Can you work these out from the model? Positions are in its coordinate system, mm. Round coordinates to 2 decimals unless told otherwise and drop trailing zeros. Write each loop counter-clockwise with the first axis right and the second up, starting at its lowest first coordinate (ties: lowest second). Pieces come first, ordered by that corner, then holes. Notation, with made-up numbers: (69.25, 15.5) -> (105.25, 15.5) arc R30 ccw to (105.25, 39.5) -> close; hole circle Ø1 at (73, 65). An arc over 180 degrees is marked (long way). Write item = value, one per line. Start each with the question number.
1) Imagine slicing it at C-C, the plane x = -71. Please give me the cut outline in (y, z), then the cut area to 3 significant figures.
2) Imagine slicing it at A-A, the plane y = 1. State how many separate pieces and enclosed holes the cut face has, then the cut area to 3 significant figures.
3) Imagine slicing it at B-B, the plane x = 10. Please give me the cut outline in (y, z).
4) If I drill on line 1 (Z direction, x = 80, y = 0.4); line 2 (X direction, y = 0.2, z = 38.5), over which ranges is the centre line in solid material (lowest first)?
5) I'm going to push flat-ended pins straight in: pin 1 (8 mm diameter, centred on x = -59, z = -58.5, fed in from -Y); pin 2 (0.6 mm diameter, centred on y = 1, z = 94, fed in from -X); pin 3 (1 mm diameter, centred on x = 0, y = 1, fed in from +Z); pin 4 (3 mm diameter, centred on x = 38.5, z = -38.5, fed in from +Y). Where does each tip first touch, or does it pass through?
from build123d import *

# Parameters (mm, degrees)
BOSS_EXTRUDE1_DEPTH     = 2
CUT_EXTRUDE1_DEPTH      = 139.261075506
CUT_EXTRUDE1_DEPTH_BACK = 139.261075506
SKETCH2_R               = 1
CHAMFER1_SIZE           = 1.5


with BuildPart() as part:
    # Sketch1 → Boss-Extrude1 (new body)
    with BuildSketch(Plane(origin=(0, 0, 0), x_dir=(1, 0, 0), z_dir=(0, 1, 0))):
        Polygon((5.75, -96.75), (61.746519787, -96.75), (61.746519787, -89.753578842), (73.246519787, -89.753578842), (73.246519787, -96.75), (96.75, -96.75), (96.75, -92.65), (91.75, -92.65), (91.75, -82.15), (96.75, -82.15), (96.75, 96.75), (23.65, 96.75), (23.65, 88.15), (-23.65, 88.15), (-23.65, 96.75), (-96.75, 96.75), (-96.75, -85.05), (-98.75, -85.05), (-98.75, -89.75), (-96.75, -89.75), (-96.75, -96.75), (-73.246519787, -96.75), (-73.246519787, -89.753578842), (-61.746519787, -89.753578842), (-61.746519787, -96.75), (-5.75, -96.75), (-5.75, -89.753578842), (5.75, -89.753578842), align=None)
    extrude(amount=BOSS_EXTRUDE1_DEPTH)

    # Sketch2 → Cut-Extrude1 (cut, two sides: drawn at the far end of the back side and taken through both)
    with BuildSketch(Plane.XZ.offset(-CUT_EXTRUDE1_DEPTH_BACK)):
        with Locations(Location((80, 80, 0), (0, 0, 270))):
            Circle(SKETCH2_R)
        with Locations(Location((-80, 80, 0), (0, 0, 270))):
            Circle(SKETCH2_R)
        with Locations(Location((-38.5, 38.5, 0), (0, 0, 270))):
            Circle(SKETCH2_R)
        with Locations(Location((38.5, 38.5, 0), (0, 0, 270))):
            Circle(SKETCH2_R)
        with Locations(Location((80, -80, 0), (0, 0, 270))):
            Circle(SKETCH2_R)
        with Locations(Location((-80, -80, 0), (0, 0, 270))):
            Circle(SKETCH2_R)
        with Locations(Location((38.5, -38.5, 0), (0, 0, 270))):
            Circle(SKETCH2_R)
        with Locations(Location((-38.5, -38.5, 0), (0, 0, 270))):
            Circle(SKETCH2_R)
    extrude(amount=CUT_EXTRUDE1_DEPTH + CUT_EXTRUDE1_DEPTH_BACK, mode=Mode.SUBTRACT)

    # Chamfer1
    chamfer1_edges = [part.edges().sort_by_distance(p)[0] for p in [
        (-80, 2, 81),
        (-38.5, 2, 39.5),
        (38.5, 2, 39.5),
        (80, 2, -79),
        (-38.5, 2, -37.5),
        (38.5, 2, -37.5),
        (-80, 2, -79),
        (80, 2, 81),
    ]]
    chamfer(chamfer1_edges, length=CHAMFER1_SIZE)


solid = part.part
Reported:
q1.outline = (0, -96.75) -> (2, -96.75) -> (2, 89.75) -> (0, 89.75) -> close
q1.area = 373 mm²
q2.separate_pieces = 1
q2.enclosed_holes = 8
q2.area = 36,700 mm²
q3.outline = (0, -88.15) -> (2, -88.15) -> (2, 96.75) -> (0, 96.75) -> close
q4.line_1 = -96.75 to -81, -79 to 79, 81 to 96.75
q4.line_2 = -96.75 to -39.5, -37.5 to 37.5, 39.5 to 96.75
q5.pin_1 = 0
q5.pin_2 = -96.75
q5.pin_3 = 89.75
q5.pin_4 = 1
